Design review of the part built by this model. Coordinates are the model's own, in mm. A direction names the side the tool comes from. Round coordinates to 2 decimals unless told otherwise and drop trailing zeros. Order: outer loops, then holes, each group sorted by start corner. A loop starts at its lowest first (then second) coordinate and runs counter-clockwise, first axis right, second up. Notation, with made-up numbers: (81.5, 69.5) - (105.5, 69.5) arc R14 cw to (105.5, 88.5) - close; hole circle Ø11 at (12, -19.75). An arc over 180 degrees is marked (long way). Use CSV: the item, a comma, the result in double quotes.
from build123d import *
from build123d.topology import SkipClean

# Parameters (mm, degrees)
ESQUISSE2_W                                       = 80
ESQUISSE2_H                                       = 85
PLAQUE_DEPTH                                      = 5.4
ESQUISSE15_R                                      = 22
D_GAGEMENT_ROUE_DEPTH                             = 81.678373806
D_COUPE_INF_RIEURE_DEPTH                          = 81.803217758
ESQUISSE14_R                                      = 11.05
ESQUISSE14_R_2                                    = 5.05
RENFORT_ROULEMENT_DEPTH                           = 2.4
D_COUPE_SUP_RIEURE_DEPTH                          = 81.803217758
D_GAGEMENT_AXE_6_DEPTH                            = 75.400336021
D_GAGEMENT_AXE_6_DEPTH_BACK                       = 75.400336021
ESQUISSE26_W                                      = 6.8
ESQUISSE26_H                                      = 6.8
D_GAGEMENT_START                                  = 1.4
D_GAGEMENT_DOUILLE_DEPTH                          = 19.2
R_P_TITION_LIN_AIRE1_COUNT                        = 2
R_P_TITION_LIN_AIRE1_PITCH                        = 26
MORS_D_FORMABLE_DOUILLE_DEPTH                     = 75.400336021
MORS_D_FORMABLE_DOUILLE_DEPTH_BACK                = 75.400336021
FRAISAGE_POUR_VIS_T_TE_FRAIS_E_BOMB_E_D           = 3.2
FRAISAGE_POUR_VIS_T_TE_FRAIS_E_BOMB_E_CSINK_D     = 6.92
FRAISAGE_POUR_VIS_T_TE_FRAIS_E_BOMB_E_CSINK_ANGLE = 90
ESQUISSE31_W                                      = 80
ESQUISSE31_H                                      = 35.1
ENL_V_MAT_EXTRU_1_DEPTH                           = 5.4
BOSS_EXTRU_1_DEPTH                                = 2.4
BOSS_EXTRU_3_START                                = -2
ESQUISSE34_R                                      = 3.46
ESQUISSE34_R_2                                    = 1.6
BOSS_EXTRU_3_DEPTH                                = 2


with BuildPart() as part:
    # Esquisse2 → plaque (new body)
    with BuildSketch(Plane(origin=(0, 0, 0), x_dir=(0, 0, -1), z_dir=(1, 0, 0))):
        with Locations((0, 27.5)):
            Rectangle(ESQUISSE2_W, ESQUISSE2_H)
    extrude(amount=PLAQUE_DEPTH)

    # Esquisse15 → dégagement roue (cut, through all)
    with BuildSketch(Plane.ZY.offset(-2.4)):
        with Locations((0, -12)):
            Circle(ESQUISSE15_R)
    extrude(amount=-D_GAGEMENT_ROUE_DEPTH, mode=Mode.SUBTRACT)

    # Esquisse18 → découpe_inférieure (cut, through all)
    with BuildSketch(Plane(origin=(0, 0, 0), x_dir=(0, 0, -1), z_dir=(1, 0, 0))):
        Polygon((-7.446869682, -5.5), (-40, -5.5), (-40, -15), (40, -15), (40, -5.5), (7.446869682, -5.5), align=None)
    extrude(amount=D_COUPE_INF_RIEURE_DEPTH, mode=Mode.SUBTRACT)

    # Esquisse14 → renfort_roulement (add)
    with BuildSketch(Plane(origin=(0, 0, 0), x_dir=(0, 0, -1), z_dir=(1, 0, 0))):
        with Locations((0, -12)):
            Circle(ESQUISSE14_R)
        with Locations((0, -12)):
            Circle(ESQUISSE14_R_2, mode=Mode.SUBTRACT)
    extrude(amount=RENFORT_ROULEMENT_DEPTH)

    # Esquisse20 → découpe_supérieure (cut, through all)
    with BuildSketch(Plane(origin=(0, 0, 0), x_dir=(0, 0, -1), z_dir=(1, 0, 0))):
        with BuildLine():
            Line((-40, 70), (40, 70))
            Line((40, 70), (40, 62.5))
            Line((40, 62.5), (26, 62.5))
            ThreePointArc((26, 62.5), (22.956192855, 61.466766701), (21.170370869, 58.794095226))
            Line((21.170370869, 58.794095226), (15.559208556, 37.852952387))
            ThreePointArc((15.559208556, 37.852952387), (14.666297563, 36.516616649), (13.144393991, 36))
            Line((13.144393991, 36), (-13.144393991, 36))
            ThreePointArc((-13.144393991, 36), (-14.666297563, 36.516616649), (-15.559208556, 37.852952387))
            Line((-15.559208556, 37.852952387), (-21.170370869, 58.794095226))
            ThreePointArc((-21.170370869, 58.794095226), (-22.956192855, 61.466766701), (-26, 62.5))
            Line((-26, 62.5), (-40, 62.5))
            Line((-40, 62.5), (-40, 70))
        make_face()
    extrude(amount=D_COUPE_SUP_RIEURE_DEPTH, mode=Mode.SUBTRACT)

    # Esquisse26 → dégagement axe 6 (cut, two sides: drawn at the far end of the back side and taken through both)
    with BuildSketch(Plane(origin=(0, 0, 0), x_dir=(1, 0, 0), z_dir=(0, 1, 0)).offset(-D_GAGEMENT_AXE_6_DEPTH_BACK)):
        with Locations((5.9, 31.5)):
            Rectangle(ESQUISSE26_W, ESQUISSE26_H)
        with Locations((5.9, -31.5)):
            Rectangle(ESQUISSE26_W, ESQUISSE26_H)
    extrude(amount=D_GAGEMENT_AXE_6_DEPTH + D_GAGEMENT_AXE_6_DEPTH_BACK, mode=Mode.SUBTRACT)

    # Esquisse28 → dégagement douille (cut)
    with BuildSketch(Plane(origin=(0, 0, 0), x_dir=(1, 0, 0), z_dir=(0, 1, 0)).offset(D_GAGEMENT_START)):
        Polygon((0, 35.5), (1.427864045, 35.5), (1.427864045, 37.7), (10.372135955, 37.7), (10.372135955, 25.3), (1.427864045, 25.3), (1.427864045, 27.5), (0, 27.5), align=None)
        Polygon((10.372135955, -25.3), (1.427864045, -25.3), (1.427864045, -27.5), (0, -27.5), (0, -35.5), (1.427864045, -35.5), (1.427864045, -37.7), (10.372135955, -37.7), align=None)
    d_gagement_douille = extrude(amount=D_GAGEMENT_DOUILLE_DEPTH, mode=Mode.SUBTRACT)

    # Répétition linéaire1: dégagement douille ×2
    with Locations(*[(0, i * R_P_TITION_LIN_AIRE1_PITCH, 0) for i in range(1, R_P_TITION_LIN_AIRE1_COUNT)]):
        add(d_gagement_douille, mode=Mode.SUBTRACT)

    # Esquisse19 → Mors_déformable_douille (cut, two sides: drawn at the far end of the back side and taken through both)
    with BuildSketch(Plane(origin=(0, 0, 0), x_dir=(1, 0, 0), z_dir=(0, 1, 0)).offset(-MORS_D_FORMABLE_DOUILLE_DEPTH_BACK)):
        Polygon((5.4, 40), (4.4, 40), (4.4, 24.1), (1, 24.1), (1, 23), (5.4, 23), align=None)
    extrude(amount=MORS_D_FORMABLE_DOUILLE_DEPTH + MORS_D_FORMABLE_DOUILLE_DEPTH_BACK, mode=Mode.SUBTRACT)

    # Fraisage pour vis à tête fraisée bombée fendue M31 (through all)
    with Locations(Plane.ZY):
        with Locations((18, 18), (36.7, 24), (36.7, -2), (21, 34)):
            fraisage_pour_vis_t_te_frais_e_bomb_e = CounterSinkHole(FRAISAGE_POUR_VIS_T_TE_FRAIS_E_BOMB_E_D / 2, FRAISAGE_POUR_VIS_T_TE_FRAIS_E_BOMB_E_CSINK_D / 2, counter_sink_angle=FRAISAGE_POUR_VIS_T_TE_FRAIS_E_BOMB_E_CSINK_ANGLE)

    # Esquisse31 → Enlèv. mat.-Extru.1 (cut)
    with BuildSketch(Plane(origin=(5.4, 0, 0), x_dir=(0, 0, -1), z_dir=(1, 0, 0))):
        with Locations((0, 44.95)):
            Rectangle(ESQUISSE31_W, ESQUISSE31_H)
    extrude(amount=-ENL_V_MAT_EXTRU_1_DEPTH, mode=Mode.SUBTRACT)

    # Esquisse33 → Boss.-Extru.1 (add)
    with BuildSketch(Plane(origin=(2.4, 0, 0), x_dir=(0, 0, -1), z_dir=(1, 0, 0))):
        Polygon((-8.125418007, -19.488663579), (-21.017849557, -5.5), (-8.936022605, -5.5), align=None)
        Polygon((8.125418007, -19.488663579), (21.017849557, -5.5), (8.936022605, -5.5), align=None)
    extrude(amount=-BOSS_EXTRU_1_DEPTH)

    # Symétrie4: Fraisage pour vis à tête fraisée bombée fendue M31 across plane
    add(fraisage_pour_vis_t_te_frais_e_bomb_e.mirror(Plane.XY), mode=Mode.SUBTRACT)

    # Esquisse34 → Boss.-Extru.3 (add)
    # profile 1 of 6: a face of its own
    with SkipClean():  # the faces are left unmerged after this step: merging them gives an invalid solid
        with BuildSketch(Plane.ZY.offset(BOSS_EXTRU_3_START)):
            with Locations((-36.7, 24)):
                Circle(ESQUISSE34_R)
            with Locations((-36.7, 24)):
                Circle(ESQUISSE34_R_2, mode=Mode.SUBTRACT)
        # profile 2 of 6: a face of its own
        with BuildSketch(Plane.ZY.offset(BOSS_EXTRU_3_START)):
            with Locations((-36.7, -2)):
                Circle(ESQUISSE34_R)
            with Locations((-36.7, -2)):
                Circle(ESQUISSE34_R_2, mode=Mode.SUBTRACT)
        # profile 3 of 6: a face of its own
        with BuildSketch(Plane.ZY.offset(BOSS_EXTRU_3_START)):
            with Locations((-18, 18)):
                Circle(ESQUISSE34_R)
            with Locations((-18, 18)):
                Circle(ESQUISSE34_R_2, mode=Mode.SUBTRACT)
        # profile 4 of 6: a face of its own
        with BuildSketch(Plane.ZY.offset(BOSS_EXTRU_3_START)):
            with Locations((18, 18)):
                Circle(ESQUISSE34_R)
            with Locations((18, 18)):
                Circle(ESQUISSE34_R_2, mode=Mode.SUBTRACT)
        # profile 5 of 6: a face of its own
        with BuildSketch(Plane.ZY.offset(BOSS_EXTRU_3_START)):
            with Locations((36.7, -2)):
                Circle(ESQUISSE34_R)
            with Locations((36.7, -2)):
                Circle(ESQUISSE34_R_2, mode=Mode.SUBTRACT)
        # profile 6 of 6: a face of its own
        with BuildSketch(Plane.ZY.offset(BOSS_EXTRU_3_START)):
            with Locations((36.7, 24)):
                Circle(ESQUISSE34_R)
            with Locations((36.7, 24)):
                Circle(ESQUISSE34_R_2, mode=Mode.SUBTRACT)
        extrude(amount=BOSS_EXTRU_3_DEPTH)


solid = part.part
1) The part is to be moulded in two halves that separate along Y. For faces 1 (the face through (1.217, -12.592, 14.481)), 2 (the face through (4.4, 11, -38)), 3 (the face through (3, 11, 40)), 4 (the face through (3, 27.4, 1)), say which applies: +Y half, -Y half, draft (parallel to the pull), parting line (faces both ways), or undercut.
Data:
face 1,"-Y half"
face 2,"draft"
face 3,"undercut"
face 4,"+Y half"
2) We need section D-D (z = 24). Give the boundary of the cut face in (x, y).
Data:
outline,"(0, -5.5) - (5.4, -5.5) - (5.4, 27.4) - (0, 27.4) - close"
3) Insertion check: pin 1 Ø1.9 at (y, z) = (-2, 36.7) entering from +X; pin 2 Ø2 at (x, z) = (4, 0.5) entering from -Y; pin 3 Ø1.3 at (x, y) = (3.5, 4.5) entering from -Z; pin 4 Ø5.5 at (y, z) = (24.5, -32.5) entering from +X. Each pin has a flat end and moves straight along its axis. Give the tip position at first contact, or say it passes through.
Data:
pin 1,"passes through"
pin 2,"stops at y = 9.95"
pin 3,"stops at z = -40"
pin 4,"stops at x = 4.4"
4) To check wall thickness, follow L1, parallel to Z at x = 1.7, y = 8; L2, parallel to Z at x = 2.8, y = 24; L3, parallel to Z at x = 2.05, y = 18. State the ranges of each line that lie inside material, in increasing order. Write a range as from..to.
Data:
L1,"z = -40..-37.7, -25.3..-24.1, -23..25.3, 37.7..40"
L2,"z = -40..-38.3, -35.1..-34.9, -28.1..-24.1, -23..28.1, 34.9..35.1, 38.3..40"
L3,"z = -40..-37.7, -25.3..-24.1, -23..-19.6, -16.4..16.4, 19.6..25.3, 37.7..40"
5) We need section C-C (z = -3). Give the boundary of the cut face in (x, y).
Data:
outline,"(0, -22.63) - (2.4, -22.63) - (2.4, -16.06) - (0, -16.06) - close; (0, -7.94) - (2.4, -7.94) - (2.4, 9.79) - (5.4, 9.79) - (5.4, 27.4) - (0, 27.4) - close"
6) We need section A-A (y = 13). Give the boundary of the cut face in (x, z), then the cut area to 3 significant figures.
Data:
outline,"(0, -40) - (4.4, -40) - (4.4, -37.7) - (1.43, -37.7) - (1.43, -35.5) - (0, -35.5) - close; (0, -27.5) - (1.43, -27.5) - (1.43, -25.3) - (4.4, -25.3) - (4.4, -24.1) - (1, -24.1) - (1, -23) - (5.4, -23) - (5.4, 25.3) - (1.43, 25.3) - (1.43, 27.5) - (0, 27.5) - close; (0, 35.5) - (1.43, 35.5) - (1.43, 37.7) - (5.4, 37.7) - (5.4, 40) - (0, 40) - close"
area,"302 mm2"
7) We need section B-B (y = -14). Give the boundary of the cut face in (x, z), then the cut area to 3 significant figures.
Data:
outline,"(0, -13.18) - (2.4, -13.18) - (2.4, -4.64) - (0, -4.64) - close; (0, 4.64) - (2.4, 4.64) - (2.4, 13.18) - (0, 13.18) - close"
area,"41.0 mm2"
8) For faces 5 (the face through (3, -2, -28.1)), 6 (the face through (2.4, -6, 0)), 7 (the face through (1, 11, 27.5)), 8 (the face through (1.428, 11, 37)), list the 3-axis set-ups (+Z, -Z, +X, -X, +Y, -Y) from which the entire face can be reached by the end or side of a thin tool; tool diameter is ignored.
Data:
face 5,"+X, +Y, -Y"
face 6,"+X, -Y"
face 7,"+X, -X"
face 8,"+X"
